Verification items for the finished model (mm, model axes). A direction names the side the tool comes from. Round coordinates to 2 decimals unless told otherwise and drop trailing zeros. Write each loop counter-clockwise with the first axis right and the second up, starting at its lowest first coordinate (ties: lowest second). Pieces come first, ordered by that corner, then holes. Notation, with made-up numbers: M 55.25,5.5 L 69.25,5.5 A30 cw 69.25,43.5 Z; hole C -14,83 d1. An arc over 180 degrees is marked long. Answer in a Markdown table with one row per item. Add a question column.
1. Material ranges on probe 1 along X at (y, z) = (-1.5, 0) (3 decimals); probe 2 along Y at (x, z) = (22.5, -0.25); probe 3 along X at (y, z) = (2.5, 0.75), recorded low to high.
2. Sectioned sample at D-D on z = 2.5. Record the cut outline in (x, y).
3. Sectioned sample at C-C on x = 36. Record the cut outline in (y, z).
4. Sectioned sample at B-B on z = -2.25. Record the cut outline in (x, y), plus the area to 3 significant figures.
5. Set-up check for faces 1 (the cylindrical face through (28.175, -0.683, -3.075)), 2 (the flat face through (58.438, -0.297, 3.773)): record each of +Z, -Z, +X, -X, +Y, -Y from which the full face is reachable in a straight line by a thin tool's end or side.
6. Sectioned sample at A-A on y = 0. Record the cut outline in (x, z) (3 decimals), plus the area to 3 significant figures.
7. Draft check along X on faces 3 (the flat face through (59.69, 0, 0)), 4 (the flat face through (58.438, 0.297, -3.773)), 5 (the cylindrical face through (2.24, -0.05, 0.86)), 6 (the flat face through (57.15, -3, 2)). Enter one of: pulls with the +X half, pulls with the -X half, needs draft (parallel to the pull), parting line crosses it, or undercut.
8. Go/stop test with flat-tipped pins: pin 1 Ø3.5 at (x, z) = (3.175, 0) entering from +Y; pin 2 Ø3 at (x, z) = (45.5, 3) entering from -Y; pin 3 Ø3 at (x, z) = (32.5, -2) entering from -Y. Record where each tip stops, or that it passes through.
```python
from build123d import *

# Parameters (mm, degrees)
F0_R     = 3.1496
F1_DEPTH = 59.69
F2_R     = 1.27
F3_DEPTH = 17.272
F4_R     = 3.1496
F5_DEPTH = 2.54
F6_DEPTH = 14.2494


with BuildPart() as f1:
    # F0 (on Right) → F1 (new body)
    with BuildSketch(Plane.YZ):
        Circle(F0_R)
    extrude(amount=F1_DEPTH)

    # F2 (on Front) → F3 (cut)
    with BuildSketch(Plane.XZ):
        with Locations((3.175, 0)):
            Circle(F2_R)
    extrude(amount=F3_DEPTH, mode=Mode.SUBTRACT)

    # F4 (on face) → F5 (join)
    with BuildSketch(Plane.YZ.offset(59.69)):
        Polygon((2.503989, -3.581569), (4.353724, 0.377734), (1.849735, 3.959303), (-2.503989, 3.581569), (-4.353724, -0.377734), (-1.849735, -3.959303), align=None)
        Circle(F4_R, mode=Mode.SUBTRACT)
    extrude(amount=-F5_DEPTH)

    # F2 (on Front) → F6 (cut)
    with BuildSketch(Plane.XZ):
        with Locations((3.175, 0)):
            Circle(F2_R)
    extrude(amount=-F6_DEPTH, mode=Mode.SUBTRACT)


solid = f1.part
```
Geometry check:
| question | item | result |
|---|---|---|
| 1 | probe 1 | x = 0 to 1.905, 4.445 to 59.69 |
| 1 | probe 2 | y = -3.14 to 3.14 |
| 1 | probe 3 | x = 0 to 2.15, 4.2 to 59.69 |
| 2 | outline | M 0,-1.92 L 57.15,-1.92 L 57.15,-3.01 L 59.69,-3.01 L 59.69,2.87 L 57.15,2.87 L 57.15,1.92 L 0,1.92 Z |
| 3 | outline | C 0,0 d6.3 |
| 4 | outline | M 0,-2.2 L 57.15,-2.2 L 57.15,-3.04 L 59.69,-3.04 L 59.69,3.13 L 57.15,3.13 L 57.15,2.2 L 0,2.2 Z |
| 4 | area | 268 mm2 |
| 5 | face 1 | -X |
| 5 | face 2 | +Z, +X, -X, -Y |
| 6 | outline | M 0,-3.15 L 57.15,-3.15 L 57.15,-3.799 L 59.69,-3.799 L 59.69,3.799 L 57.15,3.799 L 57.15,3.15 L 0,3.15 Z; hole C 3.175,0 d2.54 |
| 6 | area | 374 mm2 |
| 7 | face 3 | pulls with the +X half |
| 7 | face 4 | needs draft |
| 7 | face 5 | undercut |
| 7 | face 6 | pulls with the -X half |
| 8 | pin 1 | stops at y = 3.15 |
| 8 | pin 2 | stops at y = -2.77 |
| 8 | pin 3 | stops at y = -3.11 |
